CAD build for the part. Positions are in the model's coordinates, mm. Coordinates: 2 decimals unless noted, no trailing zeros. Loops run counter-clockwise (first coordinate to the right, second up) from the corner with the lowest first, then second, coordinate; pieces in that order, holes last. Notation, with made-up numbers: (66.5, -39.5) -> (102.5, -39.5) arc R20 ccw to (102.5, -20.5) -> close; hole circle Ø1 at (89, 81.5). An arc over 180 degrees is marked (long way). Write each question's results on one line, items separated by ' | '.
from build123d import *

# Parameters (mm, degrees)
MODEL_W             = 11.000175553
MODEL_H             = 10.999999163
BOSS_EXTRUDE1_DEPTH = 4.5


with BuildPart() as part:
    # Model → Boss-Extrude1 (new body)
    with BuildSketch(Plane.XY):
        Polygon((718.025755932, -565.527754303), (718.025755932, -552.752647917), (722.525753986, -552.752647917), (722.525718708, -528.002746812), (701.325291214, -528.002746812), (701.325291214, -523.502748758), (680.125569274, -523.502748758), (680.125569274, -528.002746812), (671.075302332, -528.002746812), (671.075302332, -548.602675974), (672.325193999, -548.602675974), (672.325193999, -551.102812084), (671.075302332, -551.102812084), (671.075302332, -553.602560139), (667.975408722, -553.602560139), (667.975408722, -551.102812084), (666.725517056, -551.102812084), (666.725517056, -548.602675974), (667.975408722, -548.602675974), (667.975408722, -528.002746812), (658.92514178, -528.002746812), (658.92514178, -523.502748758), (637.725560952, -523.502748758), (637.725560952, -528.002746812), (616.525486235, -528.002746812), (616.525486235, -552.752647917), (621.025449011, -552.752647917), (621.025449011, -565.827474303), (641.625413451, -565.827474303), (641.625413451, -564.577582637), (644.125514283, -564.577582637), (644.125514283, -565.827474303), (646.625438727, -565.827474303), (646.625438727, -568.927720691), (644.125514283, -568.927720691), (644.125514283, -570.177612357), (641.625413451, -570.177612357), (641.625413451, -568.927720691), (621.025449011, -568.927720691), (621.025449011, -582.002547077), (616.525486235, -582.002547077), (616.525486235, -603.002455683), (621.025449011, -603.002455683), (621.025449011, -624.002752344), (616.525486235, -624.002752344), (616.525486235, -645.00266095), (621.025449011, -645.00266095), (621.025449011, -666.002569556), (616.525486235, -666.002569556), (616.525486235, -687.002513439), (621.025449011, -687.002513439), (621.025449011, -708.002774823), (616.525486235, -708.002774823), (616.525486235, -729.002859818), (621.025449011, -729.002859818), (621.025449011, -750.002803701), (616.525486235, -750.002803701), (616.525486235, -771.002712307), (621.025449011, -771.002712307), (621.025449011, -784.077538693), (641.625413451, -784.077538693), (641.625413451, -782.827682304), (644.125514283, -782.827682304), (644.125514283, -784.077538693), (646.625438727, -784.077538693), (646.625438727, -787.177432303), (644.125514283, -787.177432303), (644.125514283, -788.42732397), (641.625413451, -788.42732397), (641.625413451, -787.177432303), (621.025449011, -787.177432303), (621.025449011, -800.252964244), (616.525486235, -800.252964244), (616.525486235, -825.002512572), (637.725560952, -825.002512572), (637.725560952, -829.502510626), (658.92514178, -829.502510626), (658.92514178, -825.002512572), (667.975408722, -825.002512572), (671.075302332, -825.002512572), (680.125569274, -825.002512572), (680.125569274, -829.502510626), (701.325291214, -829.502510626), (701.325291214, -825.002512572), (722.525718708, -825.002512572), (722.525753986, -800.252787855), (718.025755932, -800.252787855), (718.025755932, -787.47768147), (718.025755932, -787.177432303), (697.425438715, -787.177432303), (697.425438715, -788.42732397), (694.92569066, -788.42732397), (694.92569066, -787.177432303), (692.425237049, -787.177432303), (692.425237049, -784.077538693), (694.92569066, -784.077538693), (694.92569066, -782.827682304), (697.425438715, -782.827682304), (697.425438715, -784.077538693), (718.025755932, -784.077538693), (718.025755932, -783.777642304), (718.025755932, -771.002535918), (722.525753986, -771.002535918), (722.525753986, -750.002627312), (718.025755932, -750.002627312), (718.025755932, -729.002718707), (722.525753986, -729.002718707), (722.525753986, -708.002774823), (718.025755932, -708.002774823), (718.025755932, -687.002513439), (722.525753986, -687.002513439), (722.525753986, -666.002569556), (718.025755932, -666.002569556), (718.025755932, -645.00266095), (722.525753986, -645.00266095), (722.525753986, -624.002752344), (718.025755932, -624.002752344), (718.025755932, -603.002455683), (722.525753986, -603.002455683), (722.525753986, -582.002547077), (718.025755932, -582.002547077), (718.025755932, -569.227793469), (718.025755932, -568.927720691), (697.425438715, -568.927720691), (697.425438715, -570.177612357), (694.92569066, -570.177612357), (694.92569066, -568.927720691), (692.425237049, -568.927720691), (692.425237049, -565.827474303), (694.92569066, -565.827474303), (694.92569066, -564.577582637), (697.425438715, -564.577582637), (697.425438715, -565.827474303), (718.025755932, -565.827474303), align=None)
        with BuildLine():
            Line((715.699609821, -681.085054274), (715.699609821, -649.017765949))
            add(Edge.make_bspline(
                [(697.707943159, -649.017765949), (697.767209826, -644.081946228), (701.768344825, -640.080811229), (706.70377649, -640.080811229), (711.639913711, -640.080811229), (715.64104871, -644.081946228), (715.699609821, -649.017765949)],
                knots=[0, 0, 0, 0, 1, 1, 1, 2, 2, 2, 2], degree=3))
            Line((697.707943159, -649.017765949), (697.707943159, -681.085054274))
            add(Edge.make_bspline(
                [(697.707943159, -681.085054274), (697.707943159, -686.053223717), (701.735959825, -690.080887605), (706.70377649, -690.080887605), (711.672298711, -690.080887605), (715.699609821, -686.053223717), (715.699609821, -681.085054274)],
                knots=[0, 0, 0, 0, 1, 1, 1, 2, 2, 2, 2], degree=3))
        make_face(mode=Mode.SUBTRACT)
        with Locations((703.913939269, -588.103891659)):
            Rectangle(MODEL_W, MODEL_H, mode=Mode.SUBTRACT)
        with BuildLine():
            add(Edge.make_bspline(
                [(654.518841503, -780.523232027), (654.518841503, -772.238810362), (661.234389835, -765.523297309), (669.518811499, -765.523297309), (677.803233164, -765.523297309), (684.518746218, -772.238810362), (684.518746218, -780.523232027)],
                knots=[2, 2, 2, 2, 3, 3, 3, 4, 4, 4, 4], degree=3))
            add(Edge.make_bspline(
                [(684.518746218, -780.523232027), (684.518746218, -788.807653692), (677.803233164, -795.523202023), (669.518811499, -795.523202023), (661.234389835, -795.523202023), (654.518841503, -788.807653692), (654.518841503, -780.523232027)],
                knots=[0, 0, 0, 0, 1, 1, 1, 2, 2, 2, 2], degree=3))
        make_face(mode=Mode.SUBTRACT)
        with BuildLine():
            add(Edge.make_bspline(
                [(682.020373996, -797.456565356), (682.020373996, -795.247223968), (683.811109273, -793.456488691), (686.020133162, -793.456488691), (688.229121772, -793.456488691), (690.019892327, -795.247223968), (690.019892327, -797.456565356)],
                knots=[2, 2, 2, 2, 3, 3, 3, 4, 4, 4, 4], degree=3))
            add(Edge.make_bspline(
                [(690.019892327, -797.456565356), (690.019892327, -799.665589245), (688.229121772, -801.4566773), (686.020133162, -801.4566773), (683.811109273, -801.4566773), (682.020373996, -799.665589245), (682.020373996, -797.456565356)],
                knots=[0, 0, 0, 0, 1, 1, 1, 2, 2, 2, 2], degree=3))
        make_face(mode=Mode.SUBTRACT)
        with BuildLine():
            add(Edge.make_bspline(
                [(682.020373996, -765.353787586), (682.020373996, -763.144446198), (683.811109273, -761.353710921), (686.020133162, -761.353710921), (688.229121772, -761.353710921), (690.019892327, -763.144446198), (690.019892327, -765.353787586)],
                knots=[2, 2, 2, 2, 3, 3, 3, 4, 4, 4, 4], degree=3))
            add(Edge.make_bspline(
                [(690.019892327, -765.353787586), (690.019892327, -767.562811475), (688.229121772, -769.35389953), (686.020133162, -769.35389953), (683.811109273, -769.35389953), (682.020373996, -767.562811475), (682.020373996, -765.353787586)],
                knots=[0, 0, 0, 0, 1, 1, 1, 2, 2, 2, 2], degree=3))
        make_face(mode=Mode.SUBTRACT)
        with BuildLine():
            add(Edge.make_bspline(
                [(649.030818727, -765.353787586), (649.030818727, -763.144446198), (650.82194206, -761.353710921), (653.03124817, -761.353710921), (655.240272058, -761.353710921), (657.031007336, -763.144446198), (657.031007336, -765.353787586)],
                knots=[2, 2, 2, 2, 3, 3, 3, 4, 4, 4, 4], degree=3))
            add(Edge.make_bspline(
                [(657.031007336, -765.353787586), (657.031007336, -767.562811475), (655.240272058, -769.35389953), (653.03124817, -769.35389953), (650.82194206, -769.35389953), (649.030818727, -767.562811475), (649.030818727, -765.353787586)],
                knots=[0, 0, 0, 0, 1, 1, 1, 2, 2, 2, 2], degree=3))
        make_face(mode=Mode.SUBTRACT)
        with BuildLine():
            add(Edge.make_bspline(
                [(649.030818727, -797.456565356), (649.030818727, -795.247223968), (650.82194206, -793.456488691), (653.03124817, -793.456488691), (655.240272058, -793.456488691), (657.031007336, -795.247223968), (657.031007336, -797.456565356)],
                knots=[2, 2, 2, 2, 3, 3, 3, 4, 4, 4, 4], degree=3))
            add(Edge.make_bspline(
                [(657.031007336, -797.456565356), (657.031007336, -799.665589245), (655.240272058, -801.4566773), (653.03124817, -801.4566773), (650.82194206, -801.4566773), (649.030818727, -799.665589245), (649.030818727, -797.456565356)],
                knots=[0, 0, 0, 0, 1, 1, 1, 2, 2, 2, 2], degree=3))
        make_face(mode=Mode.SUBTRACT)
    extrude(amount=BOSS_EXTRUDE1_DEPTH)


solid = part.part
1) Slice it at B-B (z = 3.65). Count the separate pieces of the cut face and the enclosed holes in it, then the cut area to 3 significant figures.
Outcome:
separate pieces: 1 | enclosed holes: 7 | area: 28,300 mm^2
2) Drill centre lines: L1, parallel to Y at x = 697.5, z = 2.85; L2, parallel to Y at x = 627.5, z = 1; L3, parallel to X at y = -650, z = 2.45. Where is each one in solid material? Low to high. Write a range as from..to.
Outcome:
L1: y = -829.5..-787.18, -784.08..-568.93, -565.83..-523.5 | L2: y = -825..-787.18, -784.08..-568.93, -565.83..-528 | L3: x = 621.03..697.71, 715.7..718.03
3) Pin check, flat tips, straight feed: pin 1 (1.3 mm diameter, centred on y = -739, z = 2.5, fed in from +X); pin 2 (2 mm diameter, centred on x = 712.5, z = 2.5, fed in from +Y); pin 3 (2 mm diameter, centred on y = -526.5, z = 1.5, fed in from +X). Stop position of each tip, or through.
Outcome:
pin 1: stops at x = 718.03 | pin 2: stops at y = -528 | pin 3: stops at x = 701.33
4) Slice it at A-A (y = -702.5). Write the cut outline in (x, z).
Outcome:
outline: (621.03, 0) -> (718.03, 0) -> (718.03, 4.5) -> (621.03, 4.5) -> close
